Design review of the part built by this model. Coordinates are the model's own, in mm. A direction names the side the tool comes from. Coordinates: 2 decimals unless noted, no trailing zeros. Loops run counter-clockwise (first coordinate to the right, second up) from the corner with the lowest first, then second, coordinate; pieces in that order, holes last. Notation, with made-up numbers: (71.25, -8.75) - (129.25, -8.75) arc R26 ccw to (129.25, 18.25) - close; hole circle Ø11 at (15, -34.75). An arc over 180 degrees is marked (long way). Answer in a Markdown table with one row per item. Add a question column.
(1) The part is to be moulded in two halves that separate along X. For faces 6 (the face through (-11, 3, 6)), 7 (the face through (-9.927, -2.988, 4.93)), 8 (the face through (17.5, 6, 5)), 9 (the face through (15.388, 4.972, 3.201)), say which applies: released by +X, released by -X, zero draft, split by the parting line, or undercut.
(2) Clearance check with flat-ended pins moving along their axes: pin 1 (0.6 mm diameter, centred on y = 1, z = 8, fed in from -X); pin 2 (1.7 mm diameter, centred on x = -13.5, z = 5, fed in from -Y); pin 3 (6 mm diameter, centred on x = 14.5, z = 5, fed in from -Y). State where each tip first meets the part, or that it passes through.
(3) We need section A-A, the plane y = 6.5. Write out the cut boundary in (x, z) (3 decimals), plus the area to 3 significant figures.
(4) We need section C-C, the plane y = 4.5. Write out the cut boundary in (x, z) (3 decimals).
(5) For faces 1 (the face through (15.427, 4.972, 8.076)), 2 (the face through (11, 3, 6)), 3 (the face through (-6.21, 6.46, 6.06)), 4 (the face through (-0.2, 9, 1.6)), 5 (the face through (0, 1, 0)), list the 3-axis set-ups (+Z, -Z, +X, -X, +Y, -Y) from which the entire face can be reached by the end or side of a thin tool; tool diameter is ignored.
(6) We need section D-D, the plane x = 1. Write out the cut boundary in (y, z), plus the area to 3 significant figures.
(7) To check wall thickness, follow L1, parallel to Z at x = -14, y = 7.5; L2, parallel to X at y = 8.1, z = 5.65; L3, parallel to Y at x = 16, z = 9. State the ranges of each line that lie inside material, in increasing order. Write a range as [from, to].
(8) We need section B-B, the plane z = 5.65. Give the number of separate pieces and of enclosed holes in the cut face, plus the area to 3 significant figures.
from build123d import *

# Parameters (mm, degrees)
SKETCH1_W            = 35
SKETCH1_H            = 6
BOSS_EXTRUDE1_DEPTH  = 10
BOSS_EXTRUDE2_DEPTH  = 10
SKETCH4_W            = 6
SKETCH4_H            = 13.146428929
CUT_EXTRUDE1_DEPTH   = 8
CUT_EXTRUDE2_DEPTH   = 8
LPATTERN2_COUNT      = 10
LPATTERN2_PITCH      = 2
MIRROR1_COPY_1_DEPTH = 8
MIRROR1_COPY_2_DEPTH = 8
MIRROR1_COPY_3_DEPTH = 8
MIRROR1_COPY_4_DEPTH = 8
MIRROR1_COPY_5_DEPTH = 8
MIRROR1_COPY_6_DEPTH = 8
MIRROR1_COPY_7_DEPTH = 8
MIRROR1_COPY_8_DEPTH = 8
MIRROR1_COPY_9_DEPTH = 8
CUT_EXTRUDE3_DEPTH   = 25.064051894
SKETCH7_W            = 35
SKETCH7_H            = 10
BOSS_EXTRUDE3_DEPTH  = 6
SKETCH8_W            = 7.5
SKETCH8_H            = 6
CUT_EXTRUDE4_DEPTH   = 8
CUT_EXTRUDE5_DEPTH   = 4
SKETCH10_R           = 1.6
CUT_EXTRUDE6_DEPTH   = 27.462237717
CHAMFER1_SIZE        = 5


with BuildPart() as part:
    # Sketch1 → Boss-Extrude1 (new body)
    with BuildSketch(Plane.XY):
        Rectangle(SKETCH1_W, SKETCH1_H)
    extrude(amount=BOSS_EXTRUDE1_DEPTH)

    # Sketch2 → Boss-Extrude2 (add)
    with BuildSketch(Plane.XY.offset(10)):
        with BuildLine():
            Line((-17.5, -3), (17.5, -3))
            ThreePointArc((17.5, -3), (0, -10.146428929), (-17.5, -3))
        make_face()
    extrude(amount=-BOSS_EXTRUDE2_DEPTH)

    # Sketch4 → Cut-Extrude1 (cut)
    with BuildSketch(Plane.XY.offset(10)):
        with Locations((0, -3.573214465)):
            Rectangle(SKETCH4_W, SKETCH4_H)
    extrude(amount=-CUT_EXTRUDE1_DEPTH, mode=Mode.SUBTRACT)

    # Sketch5 → Cut-Extrude2 (cut)
    with BuildSketch(Plane.XY.offset(10)):
        with BuildLine():
            Line((3, 2), (3, 4))
            ThreePointArc((3, 4), (3.084360941, 3.705850588), (3.311797753, 3.501123596))
            ThreePointArc((3.311797753, 3.501123596), (3.461937846, 3.442388286), (3.619565217, 3.408543109))
            ThreePointArc((3.619565217, 3.408543109), (3.712771412, 3.358731646), (3.75, 3.259824575))
            Line((3.75, 3.259824575), (3.75, 2.740175425))
            ThreePointArc((3.75, 2.740175425), (3.712771412, 2.641268354), (3.619565217, 2.591456891))
            ThreePointArc((3.619565217, 2.591456891), (3.461937846, 2.557611714), (3.311797753, 2.498876404))
            ThreePointArc((3.311797753, 2.498876404), (3.084360941, 2.294149412), (3, 2))
        make_face()
    cut_extrude2 = extrude(amount=-CUT_EXTRUDE2_DEPTH, mode=Mode.SUBTRACT)

    # LPattern2: Cut-Extrude2 ×10
    with Locations(*[(0, -i * LPATTERN2_PITCH, 0) for i in range(1, LPATTERN2_COUNT)]):
        add(cut_extrude2, mode=Mode.SUBTRACT)

    # Mirror1: Cut-Extrude2 across plane
    add(cut_extrude2.mirror(Plane(origin=(0, 0, 0), x_dir=(0, 0, 1), z_dir=(1, 0, 0))), mode=Mode.SUBTRACT)

    # Mirror1 copy 1 sketch → Mirror1 copy 1 (cut)
    with BuildSketch(Plane(origin=(0, -2, 10), x_dir=(-1, 0, 0), z_dir=(0, 0, 1))):
        with BuildLine():
            Line((3, -2), (3, -4))
            ThreePointArc((3, -4), (3.084360941, -3.705850588), (3.311797753, -3.501123596))
            ThreePointArc((3.311797753, -3.501123596), (3.461937846, -3.442388286), (3.619565217, -3.408543109))
            ThreePointArc((3.619565217, -3.408543109), (3.712771412, -3.358731646), (3.75, -3.259824575))
            Line((3.75, -3.259824575), (3.75, -2.740175425))
            ThreePointArc((3.75, -2.740175425), (3.712771412, -2.641268354), (3.619565217, -2.591456891))
            ThreePointArc((3.619565217, -2.591456891), (3.461937846, -2.557611714), (3.311797753, -2.498876404))
            ThreePointArc((3.311797753, -2.498876404), (3.084360941, -2.294149412), (3, -2))
        make_face()
    extrude(amount=-MIRROR1_COPY_1_DEPTH, mode=Mode.SUBTRACT)

    # Mirror1 copy 2 sketch → Mirror1 copy 2 (cut)
    with BuildSketch(Plane(origin=(0, -4, 10), x_dir=(-1, 0, 0), z_dir=(0, 0, 1))):
        with BuildLine():
            Line((3, -2), (3, -4))
            ThreePointArc((3, -4), (3.084360941, -3.705850588), (3.311797753, -3.501123596))
            ThreePointArc((3.311797753, -3.501123596), (3.461937846, -3.442388286), (3.619565217, -3.408543109))
            ThreePointArc((3.619565217, -3.408543109), (3.712771412, -3.358731646), (3.75, -3.259824575))
            Line((3.75, -3.259824575), (3.75, -2.740175425))
            ThreePointArc((3.75, -2.740175425), (3.712771412, -2.641268354), (3.619565217, -2.591456891))
            ThreePointArc((3.619565217, -2.591456891), (3.461937846, -2.557611714), (3.311797753, -2.498876404))
            ThreePointArc((3.311797753, -2.498876404), (3.084360941, -2.294149412), (3, -2))
        make_face()
    extrude(amount=-MIRROR1_COPY_2_DEPTH, mode=Mode.SUBTRACT)

    # Mirror1 copy 3 sketch → Mirror1 copy 3 (cut)
    with BuildSketch(Plane(origin=(0, -6, 10), x_dir=(-1, 0, 0), z_dir=(0, 0, 1))):
        with BuildLine():
            Line((3, -2), (3, -4))
            ThreePointArc((3, -4), (3.084360941, -3.705850588), (3.311797753, -3.501123596))
            ThreePointArc((3.311797753, -3.501123596), (3.461937846, -3.442388286), (3.619565217, -3.408543109))
            ThreePointArc((3.619565217, -3.408543109), (3.712771412, -3.358731646), (3.75, -3.259824575))
            Line((3.75, -3.259824575), (3.75, -2.740175425))
            ThreePointArc((3.75, -2.740175425), (3.712771412, -2.641268354), (3.619565217, -2.591456891))
            ThreePointArc((3.619565217, -2.591456891), (3.461937846, -2.557611714), (3.311797753, -2.498876404))
            ThreePointArc((3.311797753, -2.498876404), (3.084360941, -2.294149412), (3, -2))
        make_face()
    extrude(amount=-MIRROR1_COPY_3_DEPTH, mode=Mode.SUBTRACT)

    # Mirror1 copy 4 sketch → Mirror1 copy 4 (cut)
    with BuildSketch(Plane(origin=(0, -8, 10), x_dir=(-1, 0, 0), z_dir=(0, 0, 1))):
        with BuildLine():
            Line((3, -2), (3, -4))
            ThreePointArc((3, -4), (3.084360941, -3.705850588), (3.311797753, -3.501123596))
            ThreePointArc((3.311797753, -3.501123596), (3.461937846, -3.442388286), (3.619565217, -3.408543109))
            ThreePointArc((3.619565217, -3.408543109), (3.712771412, -3.358731646), (3.75, -3.259824575))
            Line((3.75, -3.259824575), (3.75, -2.740175425))
            ThreePointArc((3.75, -2.740175425), (3.712771412, -2.641268354), (3.619565217, -2.591456891))
            ThreePointArc((3.619565217, -2.591456891), (3.461937846, -2.557611714), (3.311797753, -2.498876404))
            ThreePointArc((3.311797753, -2.498876404), (3.084360941, -2.294149412), (3, -2))
        make_face()
    extrude(amount=-MIRROR1_COPY_4_DEPTH, mode=Mode.SUBTRACT)

    # Mirror1 copy 5 sketch → Mirror1 copy 5 (cut)
    with BuildSketch(Plane(origin=(0, -10, 10), x_dir=(-1, 0, 0), z_dir=(0, 0, 1))):
        with BuildLine():
            Line((3, -2), (3, -4))
            ThreePointArc((3, -4), (3.084360941, -3.705850588), (3.311797753, -3.501123596))
            ThreePointArc((3.311797753, -3.501123596), (3.461937846, -3.442388286), (3.619565217, -3.408543109))
            ThreePointArc((3.619565217, -3.408543109), (3.712771412, -3.358731646), (3.75, -3.259824575))
            Line((3.75, -3.259824575), (3.75, -2.740175425))
            ThreePointArc((3.75, -2.740175425), (3.712771412, -2.641268354), (3.619565217, -2.591456891))
            ThreePointArc((3.619565217, -2.591456891), (3.461937846, -2.557611714), (3.311797753, -2.498876404))
            ThreePointArc((3.311797753, -2.498876404), (3.084360941, -2.294149412), (3, -2))
        make_face()
    extrude(amount=-MIRROR1_COPY_5_DEPTH, mode=Mode.SUBTRACT)

    # Mirror1 copy 6 sketch → Mirror1 copy 6 (cut)
    with BuildSketch(Plane(origin=(0, -12, 10), x_dir=(-1, 0, 0), z_dir=(0, 0, 1))):
        with BuildLine():
            Line((3, -2), (3, -4))
            ThreePointArc((3, -4), (3.084360941, -3.705850588), (3.311797753, -3.501123596))
            ThreePointArc((3.311797753, -3.501123596), (3.461937846, -3.442388286), (3.619565217, -3.408543109))
            ThreePointArc((3.619565217, -3.408543109), (3.712771412, -3.358731646), (3.75, -3.259824575))
            Line((3.75, -3.259824575), (3.75, -2.740175425))
            ThreePointArc((3.75, -2.740175425), (3.712771412, -2.641268354), (3.619565217, -2.591456891))
            ThreePointArc((3.619565217, -2.591456891), (3.461937846, -2.557611714), (3.311797753, -2.498876404))
            ThreePointArc((3.311797753, -2.498876404), (3.084360941, -2.294149412), (3, -2))
        make_face()
    extrude(amount=-MIRROR1_COPY_6_DEPTH, mode=Mode.SUBTRACT)

    # Mirror1 copy 7 sketch → Mirror1 copy 7 (cut)
    with BuildSketch(Plane(origin=(0, -14, 10), x_dir=(-1, 0, 0), z_dir=(0, 0, 1))):
        with BuildLine():
            Line((3, -2), (3, -4))
            ThreePointArc((3, -4), (3.084360941, -3.705850588), (3.311797753, -3.501123596))
            ThreePointArc((3.311797753, -3.501123596), (3.461937846, -3.442388286), (3.619565217, -3.408543109))
            ThreePointArc((3.619565217, -3.408543109), (3.712771412, -3.358731646), (3.75, -3.259824575))
            Line((3.75, -3.259824575), (3.75, -2.740175425))
            ThreePointArc((3.75, -2.740175425), (3.712771412, -2.641268354), (3.619565217, -2.591456891))
            ThreePointArc((3.619565217, -2.591456891), (3.461937846, -2.557611714), (3.311797753, -2.498876404))
            ThreePointArc((3.311797753, -2.498876404), (3.084360941, -2.294149412), (3, -2))
        make_face()
    extrude(amount=-MIRROR1_COPY_7_DEPTH, mode=Mode.SUBTRACT)

    # Mirror1 copy 8 sketch → Mirror1 copy 8 (cut)
    with BuildSketch(Plane(origin=(0, -16, 10), x_dir=(-1, 0, 0), z_dir=(0, 0, 1))):
        with BuildLine():
            Line((3, -2), (3, -4))
            ThreePointArc((3, -4), (3.084360941, -3.705850588), (3.311797753, -3.501123596))
            ThreePointArc((3.311797753, -3.501123596), (3.461937846, -3.442388286), (3.619565217, -3.408543109))
            ThreePointArc((3.619565217, -3.408543109), (3.712771412, -3.358731646), (3.75, -3.259824575))
            Line((3.75, -3.259824575), (3.75, -2.740175425))
            ThreePointArc((3.75, -2.740175425), (3.712771412, -2.641268354), (3.619565217, -2.591456891))
            ThreePointArc((3.619565217, -2.591456891), (3.461937846, -2.557611714), (3.311797753, -2.498876404))
            ThreePointArc((3.311797753, -2.498876404), (3.084360941, -2.294149412), (3, -2))
        make_face()
    extrude(amount=-MIRROR1_COPY_8_DEPTH, mode=Mode.SUBTRACT)

    # Mirror1 copy 9 sketch → Mirror1 copy 9 (cut)
    with BuildSketch(Plane(origin=(0, -18, 10), x_dir=(-1, 0, 0), z_dir=(0, 0, 1))):
        with BuildLine():
            Line((3, -2), (3, -4))
            ThreePointArc((3, -4), (3.084360941, -3.705850588), (3.311797753, -3.501123596))
            ThreePointArc((3.311797753, -3.501123596), (3.461937846, -3.442388286), (3.619565217, -3.408543109))
            ThreePointArc((3.619565217, -3.408543109), (3.712771412, -3.358731646), (3.75, -3.259824575))
            Line((3.75, -3.259824575), (3.75, -2.740175425))
            ThreePointArc((3.75, -2.740175425), (3.712771412, -2.641268354), (3.619565217, -2.591456891))
            ThreePointArc((3.619565217, -2.591456891), (3.461937846, -2.557611714), (3.311797753, -2.498876404))
            ThreePointArc((3.311797753, -2.498876404), (3.084360941, -2.294149412), (3, -2))
        make_face()
    extrude(amount=-MIRROR1_COPY_9_DEPTH, mode=Mode.SUBTRACT)

    # Sketch6 → Cut-Extrude3 (cut, through all)
    with BuildSketch(Plane(origin=(0, 3, 0), x_dir=(1, 0, 0), z_dir=(0, 1, 0))):
        Polygon((-17.5, 0), (-12.773502692, 0), (-7, -10), (-17.5, -10), align=None)
    cut_extrude3 = extrude(amount=-CUT_EXTRUDE3_DEPTH, mode=Mode.SUBTRACT)

    # Mirror2: Cut-Extrude3 across plane
    add(cut_extrude3.mirror(Plane(origin=(0, 0, 0), x_dir=(0, 0, 1), z_dir=(1, 0, 0))), mode=Mode.SUBTRACT)

    # Sketch7 → Boss-Extrude3 (add)
    with BuildSketch(Plane(origin=(0, 3, 0), x_dir=(1, 0, 0), z_dir=(0, 1, 0))):
        with Locations((0, -5)):
            Rectangle(SKETCH7_W, SKETCH7_H)
    extrude(amount=BOSS_EXTRUDE3_DEPTH)

    # Sketch8 → Cut-Extrude4 (cut)
    with BuildSketch(Plane.XY.offset(10)):
        with Locations((0, 6)):
            Rectangle(SKETCH8_W, SKETCH8_H)
    extrude(amount=-CUT_EXTRUDE4_DEPTH, mode=Mode.SUBTRACT)

    # Sketch9 → Cut-Extrude5 (cut)
    with BuildSketch(Plane.XZ.offset(-3)):
        Polygon((16.814582562, 4.025), (16.814582562, 7.275), (14, 8.9), (11.185417438, 7.275), (11.185417438, 4.025), (14, 2.4), align=None)
    cut_extrude5 = extrude(amount=-CUT_EXTRUDE5_DEPTH, mode=Mode.SUBTRACT)

    # Mirror3: Cut-Extrude5 across plane
    add(cut_extrude5.mirror(Plane(origin=(0, 0, 0), x_dir=(0, 0, 1), z_dir=(1, 0, 0))), mode=Mode.SUBTRACT)

    # Sketch10 → Cut-Extrude6 (cut, through all)
    with BuildSketch(Plane.XZ.offset(-7)):
        with Locations(Location((14, 5.65, 0), (0, 0, 270))):
            Circle(SKETCH10_R)
    cut_extrude6 = extrude(amount=-CUT_EXTRUDE6_DEPTH, mode=Mode.SUBTRACT)

    # Mirror4: Cut-Extrude6 across plane
    add(cut_extrude6.mirror(Plane(origin=(0, 0, 0), x_dir=(0, 0, 1), z_dir=(1, 0, 0))), mode=Mode.SUBTRACT)

    # Chamfer1
    chamfer1_edges = [part.edges().sort_by_distance(p)[0] for p in [
        (-3.75, 9, 6),
        (3.75, 9, 6),
    ]]
    chamfer(chamfer1_edges, length=CHAMFER1_SIZE)


solid = part.part
Responses:
| question | item | result |
|---|---|---|
| 1 | face 6 | zero draft |
| 1 | face 7 | released by -X |
| 1 | face 8 | released by +X |
| 1 | face 9 | undercut |
| 2 | pin 1 | stops at x = -8.33 |
| 2 | pin 2 | stops at y = 7 |
| 2 | pin 3 | stops at y = 3 |
| 3 | outline | (-17.5, 0) - (17.5, 0) - (17.5, 10) - (6.25, 10) - (6.25, 2) - (-6.25, 2) - (-6.25, 10) - (-17.5, 10) - close; hole (-16.815, 4.025) - (-14, 2.4) - (-11.185, 4.025) - (-11.185, 7.275) - (-14, 8.9) - (-16.815, 7.275) - close; hole (11.185, 4.025) - (14, 2.4) - (16.815, 4.025) - (16.815, 7.275) - (14, 8.9) - (11.185, 7.275) - close |
| 3 | area | 195 mm2 |
| 4 | outline | (-17.5, 0) - (17.5, 0) - (17.5, 10) - (4.25, 10) - (4.25, 2) - (-4.25, 2) - (-4.25, 10) - (-17.5, 10) - close; hole (-16.815, 4.025) - (-14, 2.4) - (-11.185, 4.025) - (-11.185, 7.275) - (-14, 8.9) - (-16.815, 7.275) - close; hole (11.185, 4.025) - (14, 2.4) - (16.815, 4.025) - (16.815, 7.275) - (14, 8.9) - (11.185, 7.275) - close |
| 5 | face 1 | -Y |
| 5 | face 2 | +Z, +X, -Y |
| 5 | face 3 | +Z, +Y |
| 5 | face 4 | +Z, -Z, +X, -X, +Y |
| 5 | face 5 | -Z, +X, -X, +Y, -Y |
| 6 | outline | (-10.13, 0) - (9, 0) - (9, 2) - (-10.13, 2) - close |
| 6 | area | 38.3 mm2 |
| 7 | L1 | z = [0, 4.05], [7.25, 10] |
| 7 | L2 | x = [-17.5, -15.6], [-12.4, -7.85], [7.85, 12.4], [15.6, 17.5] |
| 7 | L3 | y = [3, 9] |
| 8 | separate pieces | 4 |
| 8 | enclosed holes | 0 |
| 8 | area | 232 mm2 |
